Check sheet for the modelled part. Datum: model origin and axes. Units: mm. A direction names the side the tool comes from. Round coordinates to 2 decimals unless told otherwise and drop trailing zeros. Loops run counter-clockwise (first coordinate to the right, second up) from the corner with the lowest first, then second, coordinate; pieces in that order, holes last. Notation, with made-up numbers: (86, -25.75) -> (107, -25.75) arc R24 ccw to (107, -10.75) -> close; hole circle Ø10 at (-37.5, 65). An arc over 180 degrees is marked (long way). One line per item, written item: value. Start each with the question number.
1. Cross-section at B-B on y = -16.5. Record the cut outline in (x, z).
2. Material ranges on L1, parallel to X at y = -22.5, z = 15.5; L2, parallel to Y at x = 16, z = 7; L3, parallel to X at y = -12.5, z = 10, recorded low to high.
3. Release check for a two-part mould opening along Z. For faces 1 (the face through (4, -8, 38.1)), 2 (the face through (1.016, -14.89, 31.405)), 3 (the face through (25.4, -2, 19)) record: +Z half, -Z half, draft (parallel to the pull), parting line (faces both ways), or undercut.
4. Cross-section at C-C on z = 3.5. Record the cut outline in (x, y) (3 decimals), then the cut area to 3 significant figures.
5. Cross-section at D-D on x = 4. Record the cut outline in (y, z), then the cut area to 3 significant figures.
6. Go/stop test with flat-tipped pins: pin 1 (5.5 mm diameter, centred on y = -16.07, z = 30.12, fed in from +X); pin 2 (8 mm diameter, centred on y = -22.5, z = 19.5, fed in from +X); pin 3 (2 mm diameter, centred on x = 18, z = 9, fed in from -Y); pin 4 (2 mm diameter, centred on y = -15.85, z = 8.7, fed in from -X). Record where each tip stops, or that it passes through.
7. Set-up check for faces 4 (the face through (2.004, -14, 30)), 5 (the face through (4.544, -16, 19)), 6 (the face through (2, -25.4, 19)): record each of +Z, -Z, +X, -X, +Y, -Y from which the full face is reachable in a straight line by a thin tool's end or side.
Autodesk Inventor part; units mm, degrees
ref_plane "YZ Plane" through (0, 0, 0) normal (1, 0, 0) x (0, 1, 0)
ref_plane "XZ Plane" through (0, 0, 0) normal (0, 1, 0) x (-1, 0, 0)
ref_plane "XY Plane" through (0, 0, 0) normal (0, 0, 1) x (1, 0, 0)
sketch "Sketch1" plane through (0, 0, 0) normal (0, 0, 1) x (1, 0, 0)
  line L0 (0, 0) -> (25.4, 0)
  line L1 (25.4, 0) -> (25.4, -4.0087)
  line L2 (0, -25.4) -> (0, 0)
  line L3 (4.5437, -25.4) -> (0, -25.4)
  line L4 (4.5437, -25.4) -> (4.5437, -7.1837)
  line L5 (7.7187, -4.0087) -> (25.4, -4.0087)
  arc A0 (7.7187, -4.0087) -> (4.5437, -7.1837) centre (7.7187, -7.1837) ccw
  dimension "d3" = 3.175
extrude "Extrusion1" add sketch "Sketch1" along normal blind 38.1
sketch "Sketch2" plane through (4.5437, -25.4, 0) normal (1, 0, 0) x (0, 0, -1)
  circle A0 centre (-30.1153, 9.3268) radius 1.75
  circle A1 centre (-8.7049, 9.5453) radius 1.75
  point P0 (0, 25.4)
  dimension "d6" = 3.5
  dimension "d7" = 3.5
extrude "Extrusion2" cut sketch "Sketch2" against normal blind 38.1
hole "Hole1" at (4.5437, -16.0732, 30.1153) at (4.5437, -15.8547, 8.7049) direction (-1, 0, 0) diameter 9 depth 2.54
properties part number "Gyro Mount"
Taken from the geometry:
1. outline: (0, 0) -> (4.54, 0) -> (4.54, 4.25) -> (2, 4.25) -> (2, 7.08) -> (0, 7.08) -> close; (0, 10.33) -> (2, 10.33) -> (2, 13.16) -> (4.54, 13.16) -> (4.54, 25.64) -> (2, 25.64) -> (2, 28.42) -> (0, 28.42) -> close; (0, 31.81) -> (2, 31.81) -> (2, 34.6) -> (4.54, 34.6) -> (4.54, 38.1) -> (0, 38.1) -> close
2. L1: x = 0 to 4.54
2. L2: y = -4.01 to 0
2. L3: x = 0 to 2
3. face 1: +Z half
3. face 2: undercut
3. face 3: draft
4. outline: (0, -25.4) -> (4.544, -25.4) -> (4.544, -7.184) arc R3.175 cw to (7.719, -4.009) -> (25.4, -4.009) -> (25.4, 0) -> (0, 0) -> close
4. area: 201 mm2
5. outline: (-25.4, 0) -> (0, 0) -> (0, 38.1) -> (-25.4, 38.1) -> close; hole circle Ø9 at (-16.07, 30.12); hole circle Ø9 at (-15.85, 8.7)
5. area: 841 mm2
6. pin 1: stops at x = 2
6. pin 2: stops at x = 4.54
6. pin 3: stops at y = -4.01
6. pin 4: passes through
7. face 4: +X
7. face 5: +Z, -Z, +X, -Y
7. face 6: +Z, -Z, +X, -X, -Y
